from build123d import *

# Parameters (mm, degrees)
SKETCH_1_R          = 3.5
SKETCH_1_R_2        = 13
EXTRUDE_2_DEPTH     = 10
SKETCH_2_R          = 13
EXTRUDE_3_DEPTH     = 15
SKETCH_3_W          = 0.517195108
SKETCH_3_H          = 18.726193104
CUT_EXTRUDE_1_DEPTH = 26
SKETCH_4_R          = 2.5
CUT_EXTRUDE_2_DEPTH = 43.740275714
CUT_EXTRUDE_3_DEPTH = 11
SKETCH_6_R          = 2.5
CUT_EXTRUDE_4_DEPTH = 21
SKETCH_8_W          = 5
SKETCH_8_H          = 30
CUT_EXTRUDE_5_DEPTH = 26.0000001
SKETCH_9_R          = 3
CUT_EXTRUDE_6_DEPTH = 10


with BuildPart() as part:
    # 草图1 → 凸台-拉伸2 (new body)
    with BuildSketch(Plane.XY):
        with BuildLine():
            Line((-35, -7), (-7.740275714, -18.44147857))
            ThreePointArc((-7.740275714, -18.44147857), (0, -20), (7.740275714, -18.44147857))
            Line((7.740275714, -18.44147857), (35, -7))
            Line((35, -7), (35, 7))
            Line((35, 7), (7.740275714, 18.44147857))
            Line((7.740275714, 18.44147857), (7.740275714, 25.44147857))
            ThreePointArc((7.740275714, 25.44147857), (0, 27.494244152), (-7.740275714, 25.44147857))
            Line((-7.740275714, 25.44147857), (-7.740275714, 18.44147857))
            Line((-7.740275714, 18.44147857), (-35, 7))
            Line((-35, 7), (-35, -7))
        make_face()
        with Locations((-28, 0)):
            Circle(SKETCH_1_R, mode=Mode.SUBTRACT)
        Circle(SKETCH_1_R_2, mode=Mode.SUBTRACT)
        with Locations((28, 0)):
            Circle(SKETCH_1_R, mode=Mode.SUBTRACT)
    extrude(amount=EXTRUDE_2_DEPTH)

    # 草图2 → 凸台-拉伸3 (add)
    with BuildSketch(Plane.XY.offset(10)):
        with BuildLine():
            Line((-7.740275714, 18.44147857), (-7.740275714, 25.44147857))
            ThreePointArc((-7.740275714, 25.44147857), (0, 27.494244152), (7.740275714, 25.44147857))
            Line((7.740275714, 25.44147857), (7.740275714, 18.44147857))
            ThreePointArc((7.740275714, 18.44147857), (0, -20), (-7.740275714, 18.44147857))
        make_face()
        Circle(SKETCH_2_R, mode=Mode.SUBTRACT)
    extrude(amount=EXTRUDE_3_DEPTH)

    # 草图3 → 切除-拉伸1 (cut, through all)
    with BuildSketch(Plane.XY.offset(25)):
        with Locations((0, 21.741202931)):
            Rectangle(SKETCH_3_W, SKETCH_3_H)
    extrude(amount=-CUT_EXTRUDE_1_DEPTH, mode=Mode.SUBTRACT)

    # 草图4 → 切除-拉伸2 (cut, through all)
    with BuildSketch(Plane(origin=(7.740275714, 0, 0), x_dir=(0, 0, -1), z_dir=(1, 0, 0))):
        with Locations((-12.5, 21.086423576)):
            Circle(SKETCH_4_R)
    extrude(amount=-CUT_EXTRUDE_2_DEPTH, mode=Mode.SUBTRACT)

    # 草图5 → 切除-拉伸3 (cut, through all)
    with BuildSketch(Plane.XY.offset(10)):
        with BuildLine():
            Line((-7.740275714, 18.44147857), (-35, 7))
            Line((-35, 7), (-35, -7))
            Line((-35, -7), (-7.740275714, -18.44147857))
            ThreePointArc((-7.740275714, -18.44147857), (-20, 0), (-7.740275714, 18.44147857))
        make_face()
        with BuildLine():
            Line((7.740275714, 18.44147857), (35, 7))
            Line((35, 7), (35, -7))
            Line((35, -7), (7.740275714, -18.44147857))
            ThreePointArc((7.740275714, -18.44147857), (20, 0), (7.740275714, 18.44147857))
        make_face()
    extrude(amount=-CUT_EXTRUDE_3_DEPTH, mode=Mode.SUBTRACT)

    # 草图6 → 切除-拉伸4 (cut, through all)
    with BuildSketch(Plane(origin=(0, 0, 0), x_dir=(1, 0, 0), z_dir=(0, 1, 0))):
        with Locations((0, -12.5)):
            Circle(SKETCH_6_R)
    extrude(amount=-CUT_EXTRUDE_4_DEPTH, mode=Mode.SUBTRACT)

    # 草图8 → 切除-拉伸5 (cut, through all)
    with BuildSketch(Plane.XY):
        with Locations((21.5, 0)):
            Rectangle(SKETCH_8_W, SKETCH_8_H)
    extrude(amount=CUT_EXTRUDE_5_DEPTH, mode=Mode.SUBTRACT)

    # 草图9 → 切除-拉伸6 (cut)
    with BuildSketch(Plane(origin=(19, 0, 0), x_dir=(0, 0, -1), z_dir=(1, 0, 0))):
        with Locations((-12.5, 0)):
            Circle(SKETCH_9_R)
    extrude(amount=-CUT_EXTRUDE_6_DEPTH, mode=Mode.SUBTRACT)


solid = part.part
Read the model definition and answer for the solid it produces. Units are mm, in the model's axes. A direction names the side the tool comes from. Round coordinates to 2 decimals unless told otherwise and drop trailing zeros. Loops run counter-clockwise (first coordinate to the right, second up) from the corner with the lowest first, then second, coordinate; pieces in that order, holes last. Notation, with made-up numbers: (48.25, 59.25) - (75.25, 59.25) arc R24 ccw to (75.25, 80.25) - close; hole circle Ø11 at (18.25, 22). An arc over 180 degrees is marked (long way). One line per question, with ' | ' between items. Start each with the question number.
Q1. Section C-C on y = 0 is taken. Give the vertices of the cut face in (x, z).
Q2. For a pull along Y with two mould halves and no side action, classify faces 1 (the cylindrical face through (4.052, 19.565, 14.484)), 2 (the cylindrical face through (-4.182, 26.924, 12.325)), 3 (the cylindrical face through (-11.055, 6.84, 12.325)), 4 (the flat face through (19, 1.3, 9.5)) as +Y half, -Y half, draft (parallel to the pull), parting line (faces both ways), or undercut.
Q3. Section B-B on y = -16 is taken. Give the vertices of the cut face in (x, z), plus the area to 3 significant figures.
Q4. Section D-D on z = 3.25 is taken. Give the vertices of the cut face in (x, y) (3 decimals).
Q5. Flat-ended cylindrical pins translate along their axes: pin 1 (10 mm diameter, centred on x = 7, z = 22, fed in from -Y); pin 2 (3 mm diameter, centred on y = 21.5, z = 16, fed in from -X); pin 3 (6.5 mm diameter, centred on y = 21.09, z = 12.5, fed in from -X); pin 4 (15.5 mm diameter, centred on x = 0, y = 0, fed in from -Z). Find the tip coordinate at first contact, or state that the pin passes through.
Q6. Section A-A on x = -4 is taken. Give the vertices of the cut face in (y, z).
Q7. For faces 5 (the flat face through (-7.74, 24, 12)), 6 (the flat face through (-0.259, 20, 15)), 7 (the cylindrical face through (15.9, 0.1, 15.5)), 8 (the cylindrical face through (-0.54, -16.33, 14.94)), 9 (the flat face through (7.74, 24, 12)), determine the directions among +Z, -Z, +X, -X, +Y, -Y from which every point of the face is accessible in a straight line to the end or side of a thin tool.
Q8. Find the intervals of material crossed by L1, parallel to X at y = 8, z = 14; L2, parallel to X at y = 7.5, z = 8.75; L3, parallel to Y at x = 2, z = 12.5, in increasing order.
Established:
1) outline: (-20, 0) - (-13, 0) - (-13, 25) - (-20, 25) - close; (13, 0) - (19, 0) - (19, 9.5) - (13, 9.5) - close; (13, 15.5) - (19, 15.5) - (19, 25) - (13, 25) - close
2) face 1: undercut | face 2: +Y half | face 3: undercut | face 4: draft
3) outline: (-12, 0) - (12, 0) - (12, 25) - (-12, 25) - close; hole circle Ø5 at (0, 12.5) | area: 580 mm²
4) outline: (-7.74, 18.441) arc R20 ccw (long way) to (19, -6.245) - (19, 6.245) arc R20 ccw to (7.74, 18.441) - (7.74, 25.441) arc R15.619 ccw to (0.259, 27.492) - (0.259, 12.997) arc R13 cw (long way) to (-0.259, 12.997) - (-0.259, 27.492) arc R15.619 ccw to (-7.74, 25.441) - close
5) pin 1: y = -19.9 | pin 2: x = -7.74 | pin 3: x = -9.04 | pin 4: through
6) outline: (-19.6, 0) - (-12.37, 0) - (-12.37, 25) - (-19.6, 25) - close; (12.37, 0) - (26.97, 0) - (26.97, 25) - (12.37, 25) - close; hole circle Ø5 at (21.09, 12.5)
7) face 5: +Z, -Z, -X, +Y | face 6: +Z, -Z, +Y | face 7: +X | face 8: -Y | face 9: +Z, -Z, +X, +Y
8) L1: -18.33 to -10.25, 10.25 to 18.33 | L2: -18.54 to -10.62, 10.62 to 18.54 | L3: 12.85 to 18.59, 23.59 to 27.37
